```python
from build123d import *

# Parameters (mm, degrees)
F0_W     = 1422.4
F0_H     = 146.05
F1_DEPTH = 581.025
F3_DEPTH = 565.15


with BuildPart() as f1:
    # F0 (on Front) → F1 (new body)
    with BuildSketch(Plane.XZ):
        with Locations((711.2, 73.025)):
            Rectangle(F0_W, F0_H)
    extrude(amount=F1_DEPTH)

    # F2 (on face) → F3 (cut)
    with BuildSketch(Plane.XZ.offset(581.025)):
        Polygon((104.775, 120.65), (19.05, 120.65), (19.05, 19.05), (342.9, 19.05), (342.9, 120.65), (257.175, 120.65), (252.9416666667, 118.11), (340.36, 118.11), (340.36, 21.59), (21.59, 21.59), (21.59, 118.11), (109.0083333333, 118.11), align=None)
        Polygon((361.95, 120.65), (361.95, 19.05), (1060.45, 19.05), (1060.45, 120.65), (974.725, 120.65), (970.4916666667, 118.11), (1057.91, 118.11), (1057.91, 21.59), (364.49, 21.59), (364.49, 118.11), (451.9083333333, 118.11), (447.675, 120.65), align=None)
        Polygon((1165.225, 120.65), (1079.5, 120.65), (1079.5, 19.05), (1403.35, 19.05), (1403.35, 120.65), (1317.625, 120.65), (1313.3916666667, 118.11), (1400.81, 118.11), (1400.81, 21.59), (1082.04, 21.59), (1082.04, 118.11), (1169.4583333333, 118.11), align=None)
        Polygon((1317.625, 120.65), (1165.225, 120.65), (1169.4583333333, 118.11), (1313.3916666667, 118.11), align=None)
        Polygon((1313.3916666667, 118.11), (1169.4583333333, 118.11), (1196.975, 101.6), (1285.875, 101.6), align=None)
        Polygon((970.4916666667, 118.11), (451.9083333333, 118.11), (479.425, 101.6), (942.975, 101.6), align=None)
        Polygon((974.725, 120.65), (447.675, 120.65), (451.9083333333, 118.11), (970.4916666667, 118.11), align=None)
        Polygon((257.175, 120.65), (104.775, 120.65), (109.0083333333, 118.11), (252.9416666667, 118.11), align=None)
        Polygon((252.9416666667, 118.11), (109.0083333333, 118.11), (136.525, 101.6), (225.425, 101.6), align=None)
    extrude(amount=-F3_DEPTH, mode=Mode.SUBTRACT)


solid = f1.part
```
Geometry: final body of the model. Coordinates: model frame, mm. Coordinates: 2 decimals unless noted, no trailing zeros. Loops run counter-clockwise (first coordinate to the right, second up) from the corner with the lowest first, then second, coordinate; pieces in that order, holes last. Notation, with made-up numbers: M 59,-17.75 L 106,-17.75 A23 ccw 106,5.25 Z; hole C 30.5,25.5 d9. An arc over 180 degrees is marked long. Put each result on its own line as item: value.
(1) Cut plane C-C on x = 286. Return the cut outline in (y, z) (3 decimals), then the cut area to 3 significant figures.
Answer sheet:
outline: M -581.025,0 L 0,0 L 0,146.05 L -581.025,146.05 L -581.025,120.65 L -15.875,120.65 L -15.875,118.11 L -581.025,118.11 L -581.025,21.59 L -15.875,21.59 L -15.875,19.05 L -581.025,19.05 Z
area: 82,000 mm^2
(2) Cut plane A-A on y = -288. State how many separate pieces and enclosed holes the cut face has, then the cut area to 3 significant figures.
Answer sheet:
separate pieces: 4
enclosed holes: 3
area: 187,000 mm^2
(3) Cut plane B-B on x = 794.5. Return the cut outline in (y, z) (3 decimals).
Answer sheet:
outline: M -581.025,0 L 0,0 L 0,146.05 L -581.025,146.05 L -581.025,120.65 L -15.875,120.65 L -15.875,101.6 L -581.025,101.6 L -581.025,21.59 L -15.875,21.59 L -15.875,19.05 L -581.025,19.05 Z
(4) Draft query along Z for faces 1 (the face through (708, -302, 101.6)), 2 (the face through (708, -581.025, 122)), 3 (the face through (701, -286, 146.05)). Return one class per face: pulls with the +Z half, pulls with the -Z half, needs draft (parallel to the pull), parting line crosses it, or undercut.
Answer sheet:
face 1: undercut
face 2: needs draft
face 3: pulls with the +Z half
(5) Material intervals for probe 1 along Z at (x, y) = (904, -314); probe 2 along Z at (x, y) = (333, -494); probe 3 along Y at (x, z) = (954, 119) (3 decimals), sorted ascending.
Answer sheet:
probe 1: z = 0 to 19.05, 21.59 to 101.6, 120.65 to 146.05
probe 2: z = 0 to 19.05, 21.59 to 118.11, 120.65 to 146.05
probe 3: y = -15.875 to 0
